CAD build for the part. Positions are in the model's coordinates, mm. Face numbers are marked on the shaded views. A direction names the side the tool comes from. Round coordinates to 2 decimals unless told otherwise and drop trailing zeros. Order: outer loops, then holes, each group sorted by start corner. A loop starts at its lowest first (then second) coordinate and runs counter-clockwise, first axis right, second up. Notation, with made-up numbers: M 26,5.5 L 69,5.5 A22 ccw 69,28.5 Z; hole C -31,67 d4. An arc over 180 degrees is marked long. Put each result on its own line as item: value.
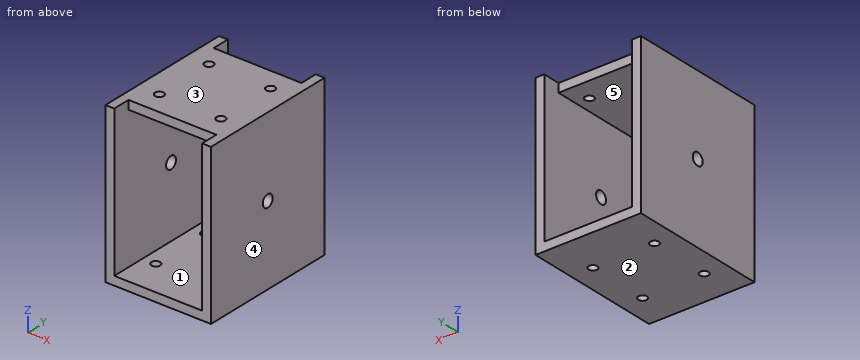
```python
from build123d import *

# Parameters (mm, degrees)
SKETCH1_W           = 60
SKETCH1_H           = 80
BOSS_EXTRUDE1_DEPTH = 80
SKETCH2_W           = 50
SKETCH2_H           = 75
CUT_EXTRUDE1_DEPTH  = 80
SKETCH3_R           = 2.5
CUT_EXTRUDE2_DEPTH  = 60
SKETCH4_R           = 3.5
CUT_EXTRUDE3_DEPTH  = 80
SKETCH5_W           = 5
SKETCH5_H           = 80
BOSS_EXTRUDE2_DEPTH = 5
SKETCH6_W           = 60
SKETCH6_H           = 80
BOSS_EXTRUDE3_DEPTH = 5
SKETCH7_R           = 2.5
CUT_EXTRUDE4_DEPTH  = 5
SKETCH8_W           = 50
SKETCH8_H           = 10
CUT_EXTRUDE5_DEPTH  = 5


with BuildPart() as part:
    # Sketch1 → Boss-Extrude1 (new body)
    with BuildSketch(Plane.XY):
        Rectangle(SKETCH1_W, SKETCH1_H)
    extrude(amount=BOSS_EXTRUDE1_DEPTH)

    # Sketch2 → Cut-Extrude1 (cut)
    with BuildSketch(Plane(origin=(0, 40, 0), x_dir=(1, 0, 0), z_dir=(0, 1, 0))):
        with Locations((0, -42.5)):
            Rectangle(SKETCH2_W, SKETCH2_H)
    extrude(amount=-CUT_EXTRUDE1_DEPTH, mode=Mode.SUBTRACT)

    # Sketch3 → Cut-Extrude2 (cut)
    with BuildSketch(Plane(origin=(0, 0, 0), x_dir=(-1, 0, 0), z_dir=(0, 0, -1))):
        with Locations((-17.5, 15)):
            Circle(SKETCH3_R)
        with Locations((17.5, 15)):
            Circle(SKETCH3_R)
        with Locations((-17.5, -20)):
            Circle(SKETCH3_R)
        with Locations((17.5, -20)):
            Circle(SKETCH3_R)
    extrude(amount=-CUT_EXTRUDE2_DEPTH, mode=Mode.SUBTRACT)

    # Sketch4 → Cut-Extrude3 (cut)
    with BuildSketch(Plane(origin=(30, 0, 0), x_dir=(0, 0, -1), z_dir=(1, 0, 0))):
        with Locations((-45, 0)):
            Circle(SKETCH4_R)
    extrude(amount=-CUT_EXTRUDE3_DEPTH, mode=Mode.SUBTRACT)

    # Sketch5 → Boss-Extrude2 (add)
    with BuildSketch(Plane.XY.offset(80)):
        with Locations((-27.5, 0)):
            Rectangle(SKETCH5_W, SKETCH5_H)
        with Locations((27.5, 0)):
            Rectangle(SKETCH5_W, SKETCH5_H)
    extrude(amount=BOSS_EXTRUDE2_DEPTH)

    # Sketch6 → Boss-Extrude3 (add)
    with BuildSketch(Plane.XY.offset(85)):
        Rectangle(SKETCH6_W, SKETCH6_H)
    extrude(amount=BOSS_EXTRUDE3_DEPTH)

    # Sketch7 → Cut-Extrude4 (cut)
    with BuildSketch(Plane.XY.offset(90)):
        with Locations((-17.5, 17.5)):
            Circle(SKETCH7_R)
        with Locations((17.5, 17.5)):
            Circle(SKETCH7_R)
        with Locations((17.5, -17.5)):
            Circle(SKETCH7_R)
        with Locations((-17.5, -17.5)):
            Circle(SKETCH7_R)
    extrude(amount=-CUT_EXTRUDE4_DEPTH, mode=Mode.SUBTRACT)

    # Sketch8 → Cut-Extrude5 (cut)
    with BuildSketch(Plane.XY.offset(90)):
        with Locations((0, 35)):
            Rectangle(SKETCH8_W, SKETCH8_H)
        with Locations((0, -35)):
            Rectangle(SKETCH8_W, SKETCH8_H)
    extrude(amount=-CUT_EXTRUDE5_DEPTH, mode=Mode.SUBTRACT)


solid = part.part
```
Item 1: Band-saw the part on B-B on x = -4. Give the cut face in (y, z), and give its area (3 significant figures).
Answers below:
outline: M -40,0 L 40,0 L 40,5 L -40,5 Z; M -30,85 L 30,85 L 30,90 L -30,90 Z
area: 700 mm²
Item 2: Band-saw the part on C-C on y = 1.5. Give the cut face in (x, z), and give its area (3 significant figures).
Answers below:
outline: M -30,0 L 30,0 L 30,41.84 L 25,41.84 L 25,5 L -25,5 L -25,41.84 L -30,41.84 Z; M -30,48.16 L -25,48.16 L -25,85 L 25,85 L 25,48.16 L 30,48.16 L 30,90 L -30,90 Z
area: 1,340 mm²
Item 3: Band-saw the part on A-A on z = 45. Give the cut face in (x, y).
Answers below:
outline: M -30,-40 L -25,-40 L -25,-3.5 L -30,-3.5 Z; M -30,3.5 L -25,3.5 L -25,40 L -30,40 Z; M 25,-40 L 30,-40 L 30,-3.5 L 25,-3.5 Z; M 25,3.5 L 30,3.5 L 30,40 L 25,40 Z
Item 4: Tool access for the marked faces 1 and 2: list every direction of +Z, -Z, +X, -X, +Y, -Y with a clear straight run to the whole face (end or side of a thin tool).
Answers below:
face 1: +Y, -Y
face 2: -Z, +X, -X, +Y, -Y
Item 5: Probe line 1 along Y through (x, z) = (-17.5, 86.25); line 2 along X through (y, z) = (4.5, 40); line 3 along Z through (x, y) = (-13.5, -29). List the from-to ranges inside material, lowest first. Write a range as [from, to].
Answers below:
line 1: [-30, -20], [-15, 15], [20, 30]
line 2: [-30, -25], [25, 30]
line 3: [0, 5], [85, 90]
Item 6: Mould opens along Z. For the marked faces 3, 4 and 5 say: pulls with the +Z half, pulls with the -Z half, needs draft (parallel to the pull), parting line crosses it, or undercut.
Answers below:
face 3: pulls with the +Z half
face 4: needs draft
face 5: undercut
Item 7: Band-saw the part on D-D on x = -17.5. Give the cut face in (y, z).
Answers below:
outline: M -40,0 L -22.5,0 L -22.5,5 L -40,5 Z; M -30,85 L -20,85 L -20,90 L -30,90 Z; M -17.5,0 L 12.5,0 L 12.5,5 L -17.5,5 Z; M -15,85 L 15,85 L 15,90 L -15,90 Z; M 17.5,0 L 40,0 L 40,5 L 17.5,5 Z; M 20,85 L 30,85 L 30,90 L 20,90 Z
Item 8: Pin check, flat tips, straight feed: P1, Ø3, axis at x = -17.5, y = 17.5, coming from the +Z side; P2, Ø6.5, axis at y = 0, z = 45, coming from the +X side; P3, Ø1.5, axis at x = -7.5, z = 86.5, coming from the +Y side; P4, Ø3, axis at x = -17.5, y = 15, coming from the -Z side. Stop position of each tip, or through.
Answers below:
P1: z = 5
P2: through
P3: y = 30
P4: z = 85
